Can you work these out from the model? Positions are in its coordinate system, mm. A direction names the side the tool comes from. Coordinates: 2 decimals unless noted, no trailing zeros. Order: outer loops, then holes, each group sorted by start corner. A loop starts at its lowest first (then second) coordinate and runs counter-clockwise, first axis right, second up. Notation, with made-up numbers: (-24.5, -3) - (12.5, -3) arc R27 ccw to (12.5, 32) - close; hole circle Ø1 at (75.25, 36). An arc over 180 degrees is marked (long way). Use a Markdown table: item, result. Add a question column.
(1) We'd pull the mould along Z, two halves only. Please class faces 4 (the cylindrical face through (-21.373, -5.083, 5.601)), 5 (the cylindrical face through (-14.5, -0.1, 14.1)), 6 (the cylindrical face through (21.373, -5.083, 5.601)), 7 (the flat face through (0, 0, 20)): pulls with the +Z half, pulls with the -Z half, needs draft (parallel to the pull), parting line crosses it, or undercut.
(2) I want a section at D-D (y = 0.5). List the corners of the cut face in (x, z) for me (3 decimals), and give its area (3 significant figures).
(3) I want a section at C-C (z = 17.5). List the corners of the cut face in (x, y) for me (3 decimals), and give its area (3 significant figures).
(4) I want a section at B-B (z = 5). List the corners of the cut face in (x, y) for me (3 decimals).
(5) I want a section at A-A (x = 17.5). List the corners of the cut face in (y, z) for me (3 decimals).
(6) For pin 1 Ø3 at (y, z) = (3.175, 5) entering from +X (3 decimals); pin 2 Ø1.8 at (x, y) = (17.5, -0.5) entering from +Z; pin 3 Ø3 at (y, z) = (-3.175, 5) entering from -X (3 decimals), each with a flat end and sliding along its axis, tell me the tip position at first contact or that it passes through.
(7) If I drill on L1, parallel to X at y = 0, z = 17 (3 decimals); L2, parallel to X at y = -2, z = 15.25 (3 decimals); L3, parallel to Y at x = 17.5, z = 12, over which ranges is the centre line in solid material (lowest first)? Write a range as [from, to].
(8) On a 3-axis mill with a long thin cutter (end or side, diameter ignored), from which of +Z, -Z, +X, -X, +Y, -Y can I reach the whole of each face in a straight line? I mean faces 1 (the cylindrical face through (-21.37, 4.65, 6.35)), 2 (the cylindrical face through (21.37, 4.65, 6.35)), 3 (the flat face through (17, 0, 8)). Say none if no direction works.
```python
from build123d import *

# Parameters (mm, degrees)
SKETCH1_W           = 56.55
SKETCH1_H           = 12.7
BOSS_EXTRUDE1_DEPTH = 20
CUT_EXTRUDE1_DEPTH  = 12
SKETCH3_R           = 2
CUT_EXTRUDE2_DEPTH  = 14


with BuildPart() as part:
    # Sketch1 → Boss-Extrude1 (new body)
    with BuildSketch(Plane.XY):
        Rectangle(SKETCH1_W, SKETCH1_H)
    extrude(amount=BOSS_EXTRUDE1_DEPTH)

    # Sketch2 → Cut-Extrude1 (cut)
    with BuildSketch(Plane.XY.offset(20)):
        with BuildLine():
            Line((-20.5, 0), (-17.5, 0))
            Line((-17.5, 0), (-14.5, 0))
            ThreePointArc((-14.5, 0), (-17.5, 3), (-20.5, 0))
        make_face()
        with BuildLine():
            Line((-14.5, 0), (-17.5, 0))
            Line((-17.5, 0), (-20.5, 0))
            ThreePointArc((-20.5, 0), (-17.5, -3), (-14.5, 0))
        make_face()
        with BuildLine():
            ThreePointArc((20.5, 0), (17.5, 3), (14.5, 0))
            Line((14.5, 0), (17.5, 0))
            Line((17.5, 0), (20.5, 0))
        make_face()
        with BuildLine():
            Line((17.5, 0), (14.5, 0))
            ThreePointArc((14.5, 0), (17.5, -3), (20.5, 0))
            Line((20.5, 0), (17.5, 0))
        make_face()
    extrude(amount=-CUT_EXTRUDE1_DEPTH, mode=Mode.SUBTRACT)

    # Sketch3 → Cut-Extrude2 (cut)
    with BuildSketch(Plane.ZY.offset(28.275)):
        with Locations(Location((5, 3.175, 0), (0, 0, 270))):
            Circle(SKETCH3_R)
        with Locations(Location((5, -3.175, 0), (0, 0, 270))):
            Circle(SKETCH3_R)
    cut_extrude2 = extrude(amount=-CUT_EXTRUDE2_DEPTH, mode=Mode.SUBTRACT)

    # Mirror1: Cut-Extrude2 across plane
    add(cut_extrude2.mirror(Plane(origin=(0, 0, 0), x_dir=(0, 0, 1), z_dir=(1, 0, 0))), mode=Mode.SUBTRACT)


solid = part.part
```
Answers follow:
| question | item | result |
|---|---|---|
| 1 | face 4 | undercut |
| 1 | face 5 | needs draft |
| 1 | face 6 | undercut |
| 1 | face 7 | pulls with the +Z half |
| 2 | outline | (-28.275, 0) - (28.275, 0) - (28.275, 20) - (20.458, 20) - (20.458, 8) - (14.542, 8) - (14.542, 20) - (-14.542, 20) - (-14.542, 8) - (-20.458, 8) - (-20.458, 20) - (-28.275, 20) - close |
| 2 | area | 989 mm² |
| 3 | outline | (-28.275, -6.35) - (28.275, -6.35) - (28.275, 6.35) - (-28.275, 6.35) - close; hole circle Ø6 at (-17.5, 0); hole circle Ø6 at (17.5, 0) |
| 3 | area | 662 mm² |
| 4 | outline | (-28.275, -6.35) - (28.275, -6.35) - (28.275, -5.175) - (14.275, -5.175) - (14.275, -1.175) - (28.275, -1.175) - (28.275, 1.175) - (14.275, 1.175) - (14.275, 5.175) - (28.275, 5.175) - (28.275, 6.35) - (-28.275, 6.35) - (-28.275, 5.175) - (-14.275, 5.175) - (-14.275, 1.175) - (-28.275, 1.175) - (-28.275, -1.175) - (-14.275, -1.175) - (-14.275, -5.175) - (-28.275, -5.175) - close |
| 5 | outline | (-6.35, 0) - (6.35, 0) - (6.35, 20) - (3, 20) - (3, 8) - (-3, 8) - (-3, 20) - (-6.35, 20) - close; hole circle Ø4 at (-3.175, 5); hole circle Ø4 at (3.175, 5) |
| 6 | pin 1 | stops at x = 14.275 |
| 6 | pin 2 | stops at z = 8 |
| 6 | pin 3 | stops at x = -14.275 |
| 7 | L1 | x = [-28.275, -20.5], [-14.5, 14.5], [20.5, 28.275] |
| 7 | L2 | x = [-28.275, -19.736], [-15.264, 15.264], [19.736, 28.275] |
| 7 | L3 | y = [-6.35, -3], [3, 6.35] |
| 8 | face 1 | -X |
| 8 | face 2 | +X |
| 8 | face 3 | +Z |
